Design review of the part built by this model. Coordinates are the model's own, in mm. Face numbers are marked on the shaded views. A direction names the side the tool comes from. Round coordinates to 2 decimals unless told otherwise and drop trailing zeros. Loops run counter-clockwise (first coordinate to the right, second up) from the corner with the lowest first, then second, coordinate; pieces in that order, holes last. Notation, with made-up numbers: M -37.5,9 L -12.5,9 A18 cw -12.5,39 Z; hole C 64,1.25 d3. An arc over 180 degrees is marked long. Use a Markdown table: item, result.
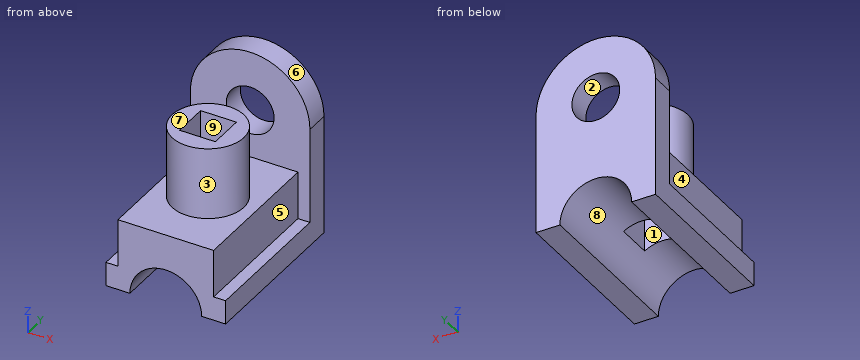
from build123d import *

# Parameters (mm, degrees)
F0_W     = 5
F0_H     = 10
F1_DEPTH = 60
F3_DEPTH = 10
F4_R     = 15
F5_DEPTH = 30
F6_W     = 15
F6_H     = 15
F7_DEPTH = 70


with BuildPart() as f1:
    # F0 (on Front) → F1 (new body)
    with BuildSketch(Plane.XZ):
        with Locations((-26.611573, 5)):
            Rectangle(F0_W, F0_H)
        with Locations((18.388427, 5)):
            Rectangle(F0_W, F0_H)
        with BuildLine():
            Line((10.888427, 0), (15.888427, 0))
            Line((15.888427, 0), (15.888427, 10))
            Line((15.888427, 10), (15.888427, 30))
            Line((15.888427, 30), (-24.111573, 30))
            Line((-24.111573, 30), (-24.111573, 10))
            Line((-24.111573, 10), (-24.111573, 0))
            Line((-24.111573, 0), (-19.111573, 0))
            ThreePointArc((-19.111573, 0), (-4.111573, 15), (10.888427, 0))
        make_face()
    extrude(amount=F1_DEPTH)

    # F2 (on face) → F3 (join)
    with BuildSketch(Plane(origin=(0, 0, 0), x_dir=(-1, 0, 0), z_dir=(0, 1, 0))):
        with BuildLine():
            Line((-20.888427, 10), (-20.888427, 0))
            Line((-20.888427, 0), (-10.888427, 0))
            ThreePointArc((-10.888427, 0), (4.111573, 15), (19.111573, 0))
            Line((19.111573, 0), (29.111573, 0))
            Line((29.111573, 0), (29.111573, 10))
            Line((29.111573, 10), (24.111573, 10))
            Line((24.111573, 10), (24.111573, 30))
            Line((24.111573, 30), (19.111573, 30))
            ThreePointArc((19.111573, 30), (4.111573, 25), (-10.888427, 30))
            Line((-10.888427, 30), (-15.888427, 30))
            Line((-15.888427, 30), (-15.888427, 10))
            Line((-15.888427, 10), (-20.888427, 10))
        make_face()
        with BuildLine():
            Line((-20.888427, 50), (-20.888427, 10))
            Line((-20.888427, 10), (-15.888427, 10))
            Line((-15.888427, 10), (-15.888427, 30))
            Line((-15.888427, 30), (-10.888427, 30))
            ThreePointArc((-10.888427, 30), (-18.249106, 38.81966), (-20.888427, 50))
        make_face()
        with BuildLine():
            Line((29.111573, 10), (29.111573, 50))
            ThreePointArc((29.111573, 50), (26.472253, 38.81966), (19.111573, 30))
            Line((19.111573, 30), (24.111573, 30))
            Line((24.111573, 30), (24.111573, 10))
            Line((24.111573, 10), (29.111573, 10))
        make_face()
        with BuildLine():
            Line((19.111573, 30), (-10.888427, 30))
            ThreePointArc((-10.888427, 30), (4.111573, 25), (19.111573, 30))
        make_face()
        with BuildLine():
            ThreePointArc((29.111573, 50), (4.111573, 75), (-20.888427, 50))
            Line((-20.888427, 50), (-5.888427, 50))
            ThreePointArc((-5.888427, 50), (4.111573, 60), (14.111573, 50))
            Line((14.111573, 50), (29.111573, 50))
        make_face()
        with BuildLine():
            Line((-5.888427, 50), (-20.888427, 50))
            ThreePointArc((-20.888427, 50), (-18.249106, 38.81966), (-10.888427, 30))
            Line((-10.888427, 30), (19.111573, 30))
            ThreePointArc((19.111573, 30), (26.472253, 38.81966), (29.111573, 50))
            Line((29.111573, 50), (14.111573, 50))
            ThreePointArc((14.111573, 50), (4.111573, 40), (-5.888427, 50))
        make_face()
    extrude(amount=F3_DEPTH)

    # F4 (on face) → F5 (join)
    with BuildSketch(Plane.XY.offset(30)):
        with Locations((-4.111573, -30)):
            Circle(F4_R)
    extrude(amount=F5_DEPTH)

    # F6 (on face) → F7 (cut)
    with BuildSketch(Plane.XY.offset(60)):
        with Locations((-4.111573, -30)):
            Rectangle(F6_W, F6_H)
    extrude(amount=-F7_DEPTH, mode=Mode.SUBTRACT)


solid = f1.part
1. Take a section at D-D on y = -2. Give the boundary of the cut face in (x, z).
Check values:
| item | result |
|---|---|
| outline | M -29.11,0 L -19.11,0 A15 cw 10.89,0 L 20.89,0 L 20.89,10 L 15.89,10 L 15.89,30 L -24.11,30 L -24.11,10 L -29.11,10 Z |
2. The part is to be moulded in two halves that separate along X. For the marked faces 6, 7, 8 and 9, say which applies: pulls with the +X half, pulls with the -X half, needs draft (parallel to the pull), parting line crosses it, or undercut.
Check values:
| item | result |
|---|---|
| face 6 | parting line crosses it |
| face 7 | needs draft |
| face 8 | undercut |
| face 9 | undercut |
3. Insertion check: pin 1 (12 mm diameter, centred on x = -10.5, y = -32.5, fed in from -Z); pin 2 (3 mm diameter, centred on x = -9.5, y = -23.5, fed in from +Z); pin 3 (6 mm diameter, centred on y = -36, z = 20.5, fed in from -X); pin 4 (2 mm diameter, centred on y = -22.5, z = 61.5, fed in from -X). Each pin has a flat end and moves straight along its axis. Give the tip position at first contact, or say it passes through.
Check values:
| item | result |
|---|---|
| pin 1 | stops at z = 8.46 |
| pin 2 | stops at z = 60 |
| pin 3 | stops at x = -24.11 |
| pin 4 | passes through |
4. Machinability: for the marked faces 1, 2, 3, 4 and 5, which of the approach directions +Z, -Z, +X, -X, +Y, -Y give a long, thin tool a straight path to every point of the face, cutting with its end or side? Answer none if there is none.
Check values:
| item | result |
|---|---|
| face 1 | +Z, -Z |
| face 2 | +Y |
| face 3 | +Z |
| face 4 | +Z, -X, -Y |
| face 5 | +Z, +X, -Y |
5. Take a section at B-B on z = 16.5. Give the boundary of the cut face in (x, y), and give its area (4 significant figures).
Check values:
| item | result |
|---|---|
| outline | M -29.11,0 L -24.11,0 L -24.11,-60 L 15.89,-60 L 15.89,0 L 20.89,0 L 20.89,10 L -29.11,10 Z; hole M -11.61,-37.5 L 3.39,-37.5 L 3.39,-22.5 L -11.61,-22.5 Z |
| area | 2,675 mm² |
6. Take a section at C-C on x = -4. Give the boundary of the cut face in (y, z).
Check values:
| item | result |
|---|---|
| outline | M -60,15 L -37.5,15 L -37.5,60 L -45,60 L -45,30 L -60,30 Z; M -22.5,15 L 10,15 L 10,40 L 0,40 L 0,30 L -15,30 L -15,60 L -22.5,60 Z; M 0,60 L 10,60 L 10,75 L 0,75 Z |
7. Take a section at A-A on y = -30. Give the boundary of the cut face in (x, z).
Check values:
| item | result |
|---|---|
| outline | M -29.11,0 L -19.11,0 A15 cw -11.61,12.99 L -11.61,60 L -19.11,60 L -19.11,30 L -24.11,30 L -24.11,10 L -29.11,10 Z; M 3.39,12.99 A15 cw 10.89,0 L 20.89,0 L 20.89,10 L 15.89,10 L 15.89,30 L 10.89,30 L 10.89,60 L 3.39,60 Z |
8. Wall thickness on line 1 along Y through (x, z) = (-8.5, 28); line 2 along Y through (x, z) = (-1, 32); line 3 along Z through (x, y) = (-12, 3.5): over which ranges is each line inside the solid? List them lowest first. Write a range as from..to.
Check values:
| item | result |
|---|---|
| line 1 | y = -60..-37.5, -22.5..10 |
| line 2 | y = -44.67..-37.5, -22.5..-15.33, 0..10 |
| line 3 | z = 12.76..43.85, 56.15..73.72 |
